Autodesk Inventor part; units mm, degrees
ref_plane "YZ Plane" through (0, 0, 0) normal (1, 0, 0) x (0, 1, 0)
ref_plane "XZ Plane" through (0, 0, 0) normal (0, 1, 0) x (-1, 0, 0)
ref_plane "XY Plane" through (0, 0, 0) normal (0, 0, 1) x (1, 0, 0)
sketch "Sketch1" plane through (0, 0, 0) normal (1, 0, 0) x (0, 1, 0)
  line L0 (-6.9148, -6.9148) -> (6.9148, 6.9148) construction
  circle A0 centre (0, 0) radius 9.779 construction
  line L1 (6.9148, -6.9148) -> (-7.1842, 7.1842) construction
  line L2 (0, 0) -> (9.779, 0) construction
  circle A1 centre (-6.9148, 6.9148) radius 1.7526
  circle A2 centre (6.9148, 6.9148) radius 1.7526
  circle A3 centre (-6.9148, -6.9148) radius 1.7526
  circle A4 centre (6.9148, -6.9148) radius 1.7526
  line L3 (-6.9148, -10.16) -> (-6.9148, 10.16) construction
  arc A5 (-5.4945, 9.8327) -> (-9.8327, 5.4945) centre (-6.9148, 6.9148) ccw
  arc A6 (-9.8327, -5.4945) -> (-5.4945, -9.8327) centre (-6.9148, -6.9148) ccw
  arc A7 (5.4945, -9.8327) -> (10.1186, -7.4317) centre (6.9148, -6.9148) ccw
  arc A8 (10.1186, 7.4317) -> (5.4945, 9.8327) centre (6.9148, 6.9148) ccw
  arc A9 (2.8448, 0.9525) -> (2.8405, -0.9652) centre (0, 0) ccw
  arc A10 (3.1276, 9.6666) -> (-3.1276, 9.6666) centre (0, 0) ccw
  line L4 (-10.16, 0) -> (16.129, 0) construction
  line L5 (16.129, 0.9525) -> (16.129, 4.7625) construction
  line L6 (16.129, -0.9652) -> (16.129, -4.7625) construction
  line L7 (16.129, 4.7625) -> (13.253, 4.7625)
  line L8 (16.129, -4.7625) -> (13.253, -4.7625)
  arc A11 (-9.6666, 3.1276) -> (-9.6666, -3.1276) centre (0, 0) ccw
  arc A12 (-3.1276, -9.6666) -> (3.1276, -9.6666) centre (0, 0) ccw
  line L9 (-10.16, -0.9652) -> (-10.114, -0.9652)
  line L10 (2.8405, -0.9652) -> (16.129, -0.9652)
  line L11 (-10.16, 0.9525) -> (-10.1153, 0.9525)
  line L12 (2.8448, 0.9525) -> (16.129, 0.9525)
  line L13 (16.129, 4.7625) -> (16.129, 0.9525)
  line L14 (16.129, -0.9652) -> (16.129, -4.7625)
  arc A13 (10.1186, 7.4317) -> (13.253, 4.7625) centre (13.253, 7.9375) ccw
  arc A14 (13.253, -4.7625) -> (10.1186, -7.4317) centre (13.253, -7.9375) ccw
  arc A15 (3.1276, 9.6666) -> (5.4945, 9.8327) centre (4.1049, 12.6875) ccw
  arc A16 (-5.4945, 9.8327) -> (-3.1276, 9.6666) centre (-4.1049, 12.6875) ccw
  arc A17 (-9.6666, 3.1276) -> (-9.8327, 5.4945) centre (-12.6875, 4.1049) ccw
  arc A18 (-9.8327, -5.4945) -> (-9.6666, -3.1276) centre (-12.6875, -4.1049) ccw
  arc A19 (-3.1276, -9.6666) -> (-5.4945, -9.8327) centre (-4.1049, -12.6875) ccw
  arc A20 (5.4945, -9.8327) -> (3.1276, -9.6666) centre (4.1049, -12.6875) ccw
  point P0 (9.3436, 4.7625)
  point P1 (9.3436, -4.7625)
  dimension "d4" = 19.558
  dimension "d6" = 3.5052
  dimension "d7" = 3.5052
  dimension "d8" = 3.5052
  dimension "d9" = 3.5052
  dimension "d11" = 6
  dimension "d12" = 26.289
  dimension "d18" = 3.175
  dimension "d19" = 3.175
extrude "Extrusion1" add sketch "Sketch1" along normal blind 6.985
sketch "Sketch2" plane through (6.985, 0, 0) normal (1, 0, 0) x (0, 0, -1)
  line L0 (0.9652, 16.129) -> (0.9652, 2.8405)
  arc A0 (-0.9525, 2.8448) -> (0.9652, 2.8405) centre (0, 0) ccw
  line L1 (-0.9525, 2.8448) -> (-0.9525, 16.129)
  arc A1 (-0.9525, 6.2782) -> (0.9652, 6.2762) centre (0, 0) ccw
  arc A2 (-0.9525, 2.8448) -> (0.9652, 2.8405) centre (0, 0) ccw
  line L2 (-0.9525, 2.8448) -> (-0.9525, 6.2782)
  line L3 (0.9652, 2.8405) -> (0.9652, 6.2762)
  dimension "d22" = 12.7
extrude "Extrusion2" add sketch "Sketch2" along normal blind 2.54
sketch "Sketch3" plane through (0, 13.253, 4.7625) normal (0, 0, 1) x (1, 0, 0)
  line L0 (0, 0) -> (6.985, 0)
  circle A0 centre (3.4925, 0) radius 1.7526
  point P0 (0, -13.253)
  dimension "d25" = 3.5052
extrude "Extrusion3" cut sketch "Sketch3" along normal mid plane 29.5275
thread "Thread1"
thread "Thread2"
chamfer "Chamfer1" distance 0.254 angle 45 39 edges at (6.985, 11.1945, 5.5202) (6.985, 8.4102, 9.7949) (6.985, 4.3271, 9.5202) (6.985, 0, 10.16) (6.985, -4.3271, 9.5202) (6.985, -9.2095, 9.2095) (6.985, -9.5202, 4.3271) (6.985, -10.16, 0) (6.985, -9.5202, -4.3271) (6.985, -9.2095, -9.2095) (6.985, -4.3271, -9.5202) (6.985, 0, -10.16) (6.985, 4.3271, -9.5202) (6.985, 8.4102, -9.7949) (6.985, 11.1945, -5.5202) (6.985, 14.691, -4.7625) (6.985, 14.691, 4.7625) (0, 11.1945, 5.5202) (0, 8.4102, 9.7949) (0, 4.3271, 9.5202) (0, 0, 10.16) (0, -4.3271, 9.5202) (0, -9.2095, 9.2095) (0, -9.5202, 4.3271) (0, -10.16, 0) (0, -9.5202, -4.3271) (0, -9.2095, -9.2095) (0, -4.3271, -9.5202) (0, 0, -10.16) (0, 4.3271, -9.5202) (0, 8.4102, -9.7949) (0, 11.1945, -5.5202) (0, 14.691, -4.7625) (0, 14.691, 4.7625) (9.525, -6.35, 0.0064) (6.985, 16.129, -2.8638) (6.985, 16.129, 2.8575) (0, 16.129, -2.8638) (0, 16.129, 2.8575)
properties part number "Clamping Hub"
Read the model definition and answer for the solid it produces. Units are mm, in the model's axes. A direction names the side the tool comes from. Coordinates: 2 decimals unless noted, no trailing zeros. Order: outer loops, then holes, each group sorted by start corner. A loop starts at its lowest first (then second) coordinate and runs counter-clockwise, first axis right, second up. Notation, with made-up numbers: (27.25, 83) -> (56.25, 83) arc R38 cw to (56.25, 122) -> close; hole circle Ø10 at (79, 25.5). An arc over 180 degrees is marked (long way). Answer as a JSON object with one key per item and string values.
1) A tool of negligible diameter and unlimited length cuts with its end or side. For faces 1 (the face through (3.45, 10.82, -5.9)), 2 (the face through (4, 9, 0.952)), 3 (the face through (6.985, 6, -4)), from which of +Z, -Z, +X, -X, +Y, -Y can it reach the whole face along a straight path? Write none if from no direction.
Model answer:
{"face 1": "-Z, +X, -X, +Y", "face 2": "+X, -X, +Y", "face 3": "+X"}
2) Each of these flat-tipped pins is pushed along its axis until it touches: pin 1 (4.5 mm diameter, centred on x = 3.49, y = 13.25, fed in from -Z); pin 2 (1.4 mm diameter, centred on x = 4.5, y = 15, fed in from +Z); pin 3 (1.4 mm diameter, centred on x = 5, y = 14.5, fed in from -Z). Where does it stop, or does it pass through?
Model answer:
{"pin 1": "stops at z = -5.7", "pin 2": "stops at z = 4.76", "pin 3": "stops at z = -4.76"}
3) A cutting plane is placed at D-D, the plane x = 6.25. Determine the outline of the cut face in (y, z), plus the area to 3 significant figures.
Model answer:
{"outline": "(-9.83, -5.49) arc R3.25 ccw to (-5.49, -9.83) arc R3.17 cw to (-3.13, -9.67) arc R10.16 ccw to (3.13, -9.67) arc R3.18 cw to (5.49, -9.83) arc R3.25 ccw to (10.12, -7.43) arc R3.17 cw to (13.25, -4.76) -> (16.13, -4.76) -> (16.13, -0.97) -> (2.84, -0.97) arc R3 cw (long way) to (2.84, 0.95) -> (16.13, 0.95) -> (16.13, 4.76) -> (13.25, 4.76) arc R3.18 cw to (10.12, 7.43) arc R3.25 ccw to (5.49, 9.83) arc R3.17 cw to (3.13, 9.67) arc R10.16 ccw to (-3.13, 9.67) arc R3.18 cw to (-5.49, 9.83) arc R3.25 ccw to (-9.83, 5.49) arc R3.17 cw to (-9.67, 3.13) arc R10.16 ccw to (-9.67, -3.13) arc R3.18 cw to start; hole circle Ø3.51 at (-6.91, -6.91); hole circle Ø3.51 at (-6.91, 6.91); hole circle Ø3.51 at (6.91, -6.91); hole circle Ø3.51 at (6.91, 6.91)", "area": "360 mm²"}
4) Consider line 1 along Z through (x, y) = (1.25, 4.25); line 2 along Y through (x, z) = (4.5, -8); line 3 along Z through (x, y) = (2, -5.5). Determine where each line is inside the solid, lowest interval first. Write a range as from..to.
Model answer:
{"line 1": "z = -9.52..-0.97, 0.95..9.52", "line 2": "y = -9.97..-8.29, -5.54..5.54, 8.29..9.97", "line 3": "z = -9.84..-7.95, -5.88..5.88, 7.95..9.84"}
5) A cutting plane is placed at A-A, the plane x = 2.5. State how many separate pieces and enclosed holes the cut face has, plus the area to 3 significant figures.
Model answer:
{"separate pieces": "3", "enclosed holes": "4", "area": "338 mm²"}
6) The mould has two halves that part along Z. Classify faces 4 (the face through (3.44, -6.11, 8.47)), 5 (the face through (3.113, 11.542, 3.152)), 6 (the face through (3.45, -0.04, 10.16)): released by +Z, released by -Z, zero draft, split by the parting line, or undercut.
Model answer:
{"face 4": "undercut", "face 5": "zero draft", "face 6": "released by +Z"}
